Geometry: final body of the model. Coordinates: model frame, mm. A direction names the side the tool comes from. Round coordinates to 2 decimals unless told otherwise and drop trailing zeros. Loops run counter-clockwise (first coordinate to the right, second up) from the corner with the lowest first, then second, coordinate; pieces in that order, holes last. Notation, with made-up numbers: M -25.5,-6 L 29.5,-6 A12 ccw 29.5,4 Z; hole C 78,-30 d8. An arc over 180 degrees is marked long. Return JSON: item names as keys, results as strings.
from build123d import *
from OCP.BRepFilletAPI import BRepFilletAPI_MakeChamfer

# Parameters (mm, degrees)
SKETCH_1_W                          = 16.59
SKETCH_1_H                          = 10.8
EXTRUDE_1_DEPTH                     = 13
FILLET_1_SIZE                       = 1
FILLET_1_SIZE_2                     = 1.5
SKETCH_2_W                          = 2
SKETCH_2_H                          = 3.5
EXTRUDE_2_DEPTH                     = 3.95
SKETCH_3_R                          = 1.5
CUT_EXTRUDE_1_DEPTH                 = 3.95
SKETCH_4_W                          = 0.5
SKETCH_4_H                          = 0.8
EXTRUDE_3_DEPTH                     = 3.5
CHAMFER_1_SIZE                      = 0.5
CHAMFER_1_SIZE2                     = 0.288675135
PATTERN_LINEAR_2_COUNT              = 4
PATTERN_LINEAR_2_PITCH              = 3.81
CHAMFER_1_OF_PATTERN_LINEAR_2_SIZE  = 0.5
CHAMFER_1_OF_PATTERN_LINEAR_2_SIZE2 = 0.288675135


with BuildPart() as part:
    # Эскиз1 → Бобышка-Вытянуть1 (new body)
    with BuildSketch(Plane.XY):
        Rectangle(SKETCH_1_W, SKETCH_1_H)
    extrude(amount=EXTRUDE_1_DEPTH)

    # Скругление1
    # an asymmetric fillet: 1.5, 1 mm, written as the material it takes off along each edge
    with BuildSketch(Plane(origin=(-12.045, -5.4, 13), x_dir=(0, 0, -1), z_dir=(1, 0, 0))) as fillet_1_piece_1:
        with BuildLine():
            Bezier((FILLET_1_SIZE, 0), (0, 0), (0, FILLET_1_SIZE_2), weights=[1, 0.707106781, 1])
            Line((0, FILLET_1_SIZE_2), (0, 0))
            Line((0, 0), (FILLET_1_SIZE, 0))
        make_face()
    extrude(amount=24.09, mode=Mode.SUBTRACT)

    # Эскиз2 → Бобышка-Вытянуть2 (add)
    with BuildSketch(Plane.XY.offset(13)):
        with Locations((5.485, 2.4)):
            Rectangle(SKETCH_2_W, SKETCH_2_H)
    extrude_2 = extrude(amount=EXTRUDE_2_DEPTH)

    # Эскиз3 → Вырез-Вытянуть1 (cut)
    with BuildSketch(Plane.XY.offset(13)):
        with Locations((6.195, -1.686021073)):
            Circle(SKETCH_3_R)
    cut_extrude_1 = extrude(amount=-CUT_EXTRUDE_1_DEPTH, mode=Mode.SUBTRACT)

    # Эскиз4 → Бобышка-Вытянуть3 (add)
    with BuildSketch(Plane(origin=(0, 0, 0), x_dir=(-1, 0, 0), z_dir=(0, 0, -1))):
        with Locations((-7.255, 2.85)):
            Rectangle(SKETCH_4_W, SKETCH_4_H)
        with Locations((-7.255, -2.15)):
            Rectangle(SKETCH_4_W, SKETCH_4_H)
    extrude_3 = extrude(amount=EXTRUDE_3_DEPTH)

    # Фаска1: one chamfer whose edges measure the first distance from different faces: ONE call of the kernel's chamfer builder (chamfer() names one face for all edges)
    chamfer_1_edges_1 = [part.edges().sort_by_distance(p)[0] for p in [
        (7.255, 3.25, -3.5),
    ]]
    chamfer_1_side_1 = [part.faces().sort_by_distance(p)[0] for p in [
        (7.255, 3.25, -1.75),
    ]]
    chamfer_1_edges_2 = [part.edges().sort_by_distance(p)[0] for p in [
        (7.255, 2.45, -3.5),
    ]]
    chamfer_1_side_2 = [part.faces().sort_by_distance(p)[0] for p in [
        (7.255, 2.45, -1.75),
    ]]
    chamfer_1_edges_3 = [part.edges().sort_by_distance(p)[0] for p in [
        (7.255, -2.55, -3.5),
    ]]
    chamfer_1_side_3 = [part.faces().sort_by_distance(p)[0] for p in [
        (7.255, -2.55, -1.75),
    ]]
    chamfer_1_edges_4 = [part.edges().sort_by_distance(p)[0] for p in [
        (7.255, -1.75, -3.5),
    ]]
    chamfer_1_side_4 = [part.faces().sort_by_distance(p)[0] for p in [
        (7.255, -1.75, -1.75),
    ]]
    chamfer_1 = BRepFilletAPI_MakeChamfer(part.part.solid().wrapped)
    for e in chamfer_1_edges_1:
        chamfer_1.Add(CHAMFER_1_SIZE, CHAMFER_1_SIZE2, e.wrapped, chamfer_1_side_1[0].wrapped)  # the first distance lies on this face
    for e in chamfer_1_edges_2:
        chamfer_1.Add(CHAMFER_1_SIZE, CHAMFER_1_SIZE2, e.wrapped, chamfer_1_side_2[0].wrapped)  # the first distance lies on this face
    for e in chamfer_1_edges_3:
        chamfer_1.Add(CHAMFER_1_SIZE, CHAMFER_1_SIZE2, e.wrapped, chamfer_1_side_3[0].wrapped)  # the first distance lies on this face
    for e in chamfer_1_edges_4:
        chamfer_1.Add(CHAMFER_1_SIZE, CHAMFER_1_SIZE2, e.wrapped, chamfer_1_side_4[0].wrapped)  # the first distance lies on this face
    add(Compound.cast(chamfer_1.Shape()), mode=Mode.REPLACE)

    # Линейный массив2: Бобышка-Вытянуть2, Вырез-Вытянуть1, Бобышка-Вытянуть3 ×4
    with Locations(*[(-i * PATTERN_LINEAR_2_PITCH, 0, 0) for i in range(1, PATTERN_LINEAR_2_COUNT)]):
        add(extrude_2)
        add(cut_extrude_1, mode=Mode.SUBTRACT)
        add(extrude_3)

    # Фаска1 of Линейный массив2: one chamfer whose edges measure the first distance from different faces: ONE call of the kernel's chamfer builder (chamfer() names one face for all edges)
    chamfer_1_of_pattern_linear_2_edges_1 = [part.edges().sort_by_distance(p)[0] for p in [
        (3.445, 3.25, -3.5),
    ]]
    chamfer_1_of_pattern_linear_2_side_1 = [part.faces().sort_by_distance(p)[0] for p in [
        (3.445, 3.25, -1.75),
    ]]
    chamfer_1_of_pattern_linear_2_edges_2 = [part.edges().sort_by_distance(p)[0] for p in [
        (3.445, 2.45, -3.5),
    ]]
    chamfer_1_of_pattern_linear_2_side_2 = [part.faces().sort_by_distance(p)[0] for p in [
        (3.445, 2.45, -1.75),
    ]]
    chamfer_1_of_pattern_linear_2_edges_3 = [part.edges().sort_by_distance(p)[0] for p in [
        (3.445, -2.55, -3.5),
    ]]
    chamfer_1_of_pattern_linear_2_side_3 = [part.faces().sort_by_distance(p)[0] for p in [
        (3.445, -2.55, -1.75),
    ]]
    chamfer_1_of_pattern_linear_2_edges_4 = [part.edges().sort_by_distance(p)[0] for p in [
        (3.445, -1.75, -3.5),
    ]]
    chamfer_1_of_pattern_linear_2_side_4 = [part.faces().sort_by_distance(p)[0] for p in [
        (3.445, -1.75, -1.75),
    ]]
    chamfer_1_of_pattern_linear_2_edges_5 = [part.edges().sort_by_distance(p)[0] for p in [
        (-0.365, 3.25, -3.5),
    ]]
    chamfer_1_of_pattern_linear_2_side_5 = [part.faces().sort_by_distance(p)[0] for p in [
        (-0.365, 3.25, -1.75),
    ]]
    chamfer_1_of_pattern_linear_2_edges_6 = [part.edges().sort_by_distance(p)[0] for p in [
        (-0.365, 2.45, -3.5),
    ]]
    chamfer_1_of_pattern_linear_2_side_6 = [part.faces().sort_by_distance(p)[0] for p in [
        (-0.365, 2.45, -1.75),
    ]]
    chamfer_1_of_pattern_linear_2_edges_7 = [part.edges().sort_by_distance(p)[0] for p in [
        (-0.365, -2.55, -3.5),
    ]]
    chamfer_1_of_pattern_linear_2_side_7 = [part.faces().sort_by_distance(p)[0] for p in [
        (-0.365, -2.55, -1.75),
    ]]
    chamfer_1_of_pattern_linear_2_edges_8 = [part.edges().sort_by_distance(p)[0] for p in [
        (-0.365, -1.75, -3.5),
    ]]
    chamfer_1_of_pattern_linear_2_side_8 = [part.faces().sort_by_distance(p)[0] for p in [
        (-0.365, -1.75, -1.75),
    ]]
    chamfer_1_of_pattern_linear_2_edges_9 = [part.edges().sort_by_distance(p)[0] for p in [
        (-4.175, 3.25, -3.5),
    ]]
    chamfer_1_of_pattern_linear_2_side_9 = [part.faces().sort_by_distance(p)[0] for p in [
        (-4.175, 3.25, -1.75),
    ]]
    chamfer_1_of_pattern_linear_2_edges_10 = [part.edges().sort_by_distance(p)[0] for p in [
        (-4.175, 2.45, -3.5),
    ]]
    chamfer_1_of_pattern_linear_2_side_10 = [part.faces().sort_by_distance(p)[0] for p in [
        (-4.175, 2.45, -1.75),
    ]]
    chamfer_1_of_pattern_linear_2_edges_11 = [part.edges().sort_by_distance(p)[0] for p in [
        (-4.175, -2.55, -3.5),
    ]]
    chamfer_1_of_pattern_linear_2_side_11 = [part.faces().sort_by_distance(p)[0] for p in [
        (-4.175, -2.55, -1.75),
    ]]
    chamfer_1_of_pattern_linear_2_edges_12 = [part.edges().sort_by_distance(p)[0] for p in [
        (-4.175, -1.75, -3.5),
    ]]
    chamfer_1_of_pattern_linear_2_side_12 = [part.faces().sort_by_distance(p)[0] for p in [
        (-4.175, -1.75, -1.75),
    ]]
    chamfer_1_of_pattern_linear_2 = BRepFilletAPI_MakeChamfer(part.part.solid().wrapped)
    for e in chamfer_1_of_pattern_linear_2_edges_1:
        chamfer_1_of_pattern_linear_2.Add(CHAMFER_1_OF_PATTERN_LINEAR_2_SIZE, CHAMFER_1_OF_PATTERN_LINEAR_2_SIZE2, e.wrapped, chamfer_1_of_pattern_linear_2_side_1[0].wrapped)  # the first distance lies on this face
    for e in chamfer_1_of_pattern_linear_2_edges_2:
        chamfer_1_of_pattern_linear_2.Add(CHAMFER_1_OF_PATTERN_LINEAR_2_SIZE, CHAMFER_1_OF_PATTERN_LINEAR_2_SIZE2, e.wrapped, chamfer_1_of_pattern_linear_2_side_2[0].wrapped)  # the first distance lies on this face
    for e in chamfer_1_of_pattern_linear_2_edges_3:
        chamfer_1_of_pattern_linear_2.Add(CHAMFER_1_OF_PATTERN_LINEAR_2_SIZE, CHAMFER_1_OF_PATTERN_LINEAR_2_SIZE2, e.wrapped, chamfer_1_of_pattern_linear_2_side_3[0].wrapped)  # the first distance lies on this face
    for e in chamfer_1_of_pattern_linear_2_edges_4:
        chamfer_1_of_pattern_linear_2.Add(CHAMFER_1_OF_PATTERN_LINEAR_2_SIZE, CHAMFER_1_OF_PATTERN_LINEAR_2_SIZE2, e.wrapped, chamfer_1_of_pattern_linear_2_side_4[0].wrapped)  # the first distance lies on this face
    for e in chamfer_1_of_pattern_linear_2_edges_5:
        chamfer_1_of_pattern_linear_2.Add(CHAMFER_1_OF_PATTERN_LINEAR_2_SIZE, CHAMFER_1_OF_PATTERN_LINEAR_2_SIZE2, e.wrapped, chamfer_1_of_pattern_linear_2_side_5[0].wrapped)  # the first distance lies on this face
    for e in chamfer_1_of_pattern_linear_2_edges_6:
        chamfer_1_of_pattern_linear_2.Add(CHAMFER_1_OF_PATTERN_LINEAR_2_SIZE, CHAMFER_1_OF_PATTERN_LINEAR_2_SIZE2, e.wrapped, chamfer_1_of_pattern_linear_2_side_6[0].wrapped)  # the first distance lies on this face
    for e in chamfer_1_of_pattern_linear_2_edges_7:
        chamfer_1_of_pattern_linear_2.Add(CHAMFER_1_OF_PATTERN_LINEAR_2_SIZE, CHAMFER_1_OF_PATTERN_LINEAR_2_SIZE2, e.wrapped, chamfer_1_of_pattern_linear_2_side_7[0].wrapped)  # the first distance lies on this face
    for e in chamfer_1_of_pattern_linear_2_edges_8:
        chamfer_1_of_pattern_linear_2.Add(CHAMFER_1_OF_PATTERN_LINEAR_2_SIZE, CHAMFER_1_OF_PATTERN_LINEAR_2_SIZE2, e.wrapped, chamfer_1_of_pattern_linear_2_side_8[0].wrapped)  # the first distance lies on this face
    for e in chamfer_1_of_pattern_linear_2_edges_9:
        chamfer_1_of_pattern_linear_2.Add(CHAMFER_1_OF_PATTERN_LINEAR_2_SIZE, CHAMFER_1_OF_PATTERN_LINEAR_2_SIZE2, e.wrapped, chamfer_1_of_pattern_linear_2_side_9[0].wrapped)  # the first distance lies on this face
    for e in chamfer_1_of_pattern_linear_2_edges_10:
        chamfer_1_of_pattern_linear_2.Add(CHAMFER_1_OF_PATTERN_LINEAR_2_SIZE, CHAMFER_1_OF_PATTERN_LINEAR_2_SIZE2, e.wrapped, chamfer_1_of_pattern_linear_2_side_10[0].wrapped)  # the first distance lies on this face
    for e in chamfer_1_of_pattern_linear_2_edges_11:
        chamfer_1_of_pattern_linear_2.Add(CHAMFER_1_OF_PATTERN_LINEAR_2_SIZE, CHAMFER_1_OF_PATTERN_LINEAR_2_SIZE2, e.wrapped, chamfer_1_of_pattern_linear_2_side_11[0].wrapped)  # the first distance lies on this face
    for e in chamfer_1_of_pattern_linear_2_edges_12:
        chamfer_1_of_pattern_linear_2.Add(CHAMFER_1_OF_PATTERN_LINEAR_2_SIZE, CHAMFER_1_OF_PATTERN_LINEAR_2_SIZE2, e.wrapped, chamfer_1_of_pattern_linear_2_side_12[0].wrapped)  # the first distance lies on this face
    add(Compound.cast(chamfer_1_of_pattern_linear_2.Shape()), mode=Mode.REPLACE)


solid = part.part
Q1. Section query C-C (z = -1). State how many separate pieces and enclosed holes the cut face has, plus the area to 3 significant figures.
Determined:
{"separate pieces": "8", "enclosed holes": "0", "area": "3.20 mm^2"}
Q2. Reachability of faces 4 (the flat face through (0, -5.4, 6)), 5 (the flat face through (2, 0.65, 15)), 6 (the flat face through (4.485, 2, 15)), 7 (the flat face through (0, 5.4, 6)), 8 (the flat face through (2, -2, 9.05)) from +Z, -Z, +X, -X, +Y, -Y: full face, straight path, thin tool, end or side. Return the list, or none.
Determined:
{"face 4": "+Z, -Z, +X, -X, -Y", "face 5": "+Z, +X, -X, -Y", "face 6": "+Z, +Y, -Y", "face 7": "+Z, -Z, +X, -X, +Y", "face 8": "+Z"}
Q3. Section query B-B (y = 1.5). Output: boundary loops of the cut face in (x, z) (3 decimals), plus the area to 3 significant figures.
Determined:
{"outline": "M -8.295,0 L 8.295,0 L 8.295,13 L 6.485,13 L 6.485,16.95 L 4.485,16.95 L 4.485,13 L 2.675,13 L 2.675,16.95 L 0.675,16.95 L 0.675,13 L -1.135,13 L -1.135,16.95 L -3.135,16.95 L -3.135,13 L -4.945,13 L -4.945,16.95 L -6.945,16.95 L -6.945,13 L -8.295,13 Z", "area": "247 mm^2"}
Q4. Pull-direction query (X, two-part tool) for faces 1 (the flat face through (5, 0.65, 15)), 2 (the flat face through (-1, -2, 9.05)), 3 (the flat face through (-6.945, 2, 15)); classes: pulls with the +X half, pulls with the -X half, needs draft (parallel to the pull), parting line crosses it, or undercut.
Determined:
{"face 1": "needs draft", "face 2": "undercut", "face 3": "pulls with the -X half"}
Q5. Material intervals for L1, parallel to X at y = 3.5, z = 14 (3 decimals); L2, parallel to Z at x = 0.75, y = 3; L3, parallel to Y at x = -2.25, z = 13.5, sorted ascending.
Determined:
{"L1": "x = -6.945 to -4.945, -3.135 to -1.135, 0.675 to 2.675, 4.485 to 6.485", "L2": "z = 0 to 16.95", "L3": "y = 0.65 to 4.15"}
Q6. Section query A-A (z = 15.5). Output: boundary loops of the cut face in (x, y) (3 decimals).
Determined:
{"outline": "M -6.945,0.65 L -4.945,0.65 L -4.945,4.15 L -6.945,4.15 Z; M -3.135,0.65 L -1.135,0.65 L -1.135,4.15 L -3.135,4.15 Z; M 0.675,0.65 L 2.675,0.65 L 2.675,4.15 L 0.675,4.15 Z; M 4.485,0.65 L 6.485,0.65 L 6.485,4.15 L 4.485,4.15 Z"}
Q7. Pin query (flat end, axial travel): pin 1 (0.6 mm diameter, centred on y = -2, z = -2, fed in from +X) (3 decimals); pin 2 (0.6 mm diameter, centred on y = -2, z = -1.5, fed in from -X) (3 decimals); pin 3 (1 mm diameter, centred on x = -2.5, z = 14, fed in from +Y); pin 4 (3 mm diameter, centred on x = -6, z = 14, fed in from +Y). Return the tip coordinate at first contact, or that it passes through.
Determined:
{"pin 1": "stops at x = 7.505", "pin 2": "stops at x = -4.425", "pin 3": "stops at y = 4.15", "pin 4": "stops at y = 5.4"}
Q8. Section query D-D (y = 0.25). Output: boundary loops of the cut face in (x, z) (3 decimals), plus the area to 3 significant figures.
Determined:
{"outline": "M -8.295,0 L 8.295,0 L 8.295,13 L -8.295,13 Z", "area": "216 mm^2"}
